Answer from the drawing. Dimensions are ordinates in mm from the lowest x, y and z of the part. A direction names the side the tool comes from. Coordinates: 2 decimals unless noted, no trailing zeros. Order: outer loops, then holes, each group sorted by start corner. A loop starts at its lowest first (then second) coordinate and runs counter-clockwise, first axis right, second up. Notation, with made-up numbers: M 84,11 L 112,11 A7 ccw 112,23 Z; hole C 32.5,-0.5 d3. An arc over 180 degrees is marked long. Write each question's results on one line, items separated by ' | '.
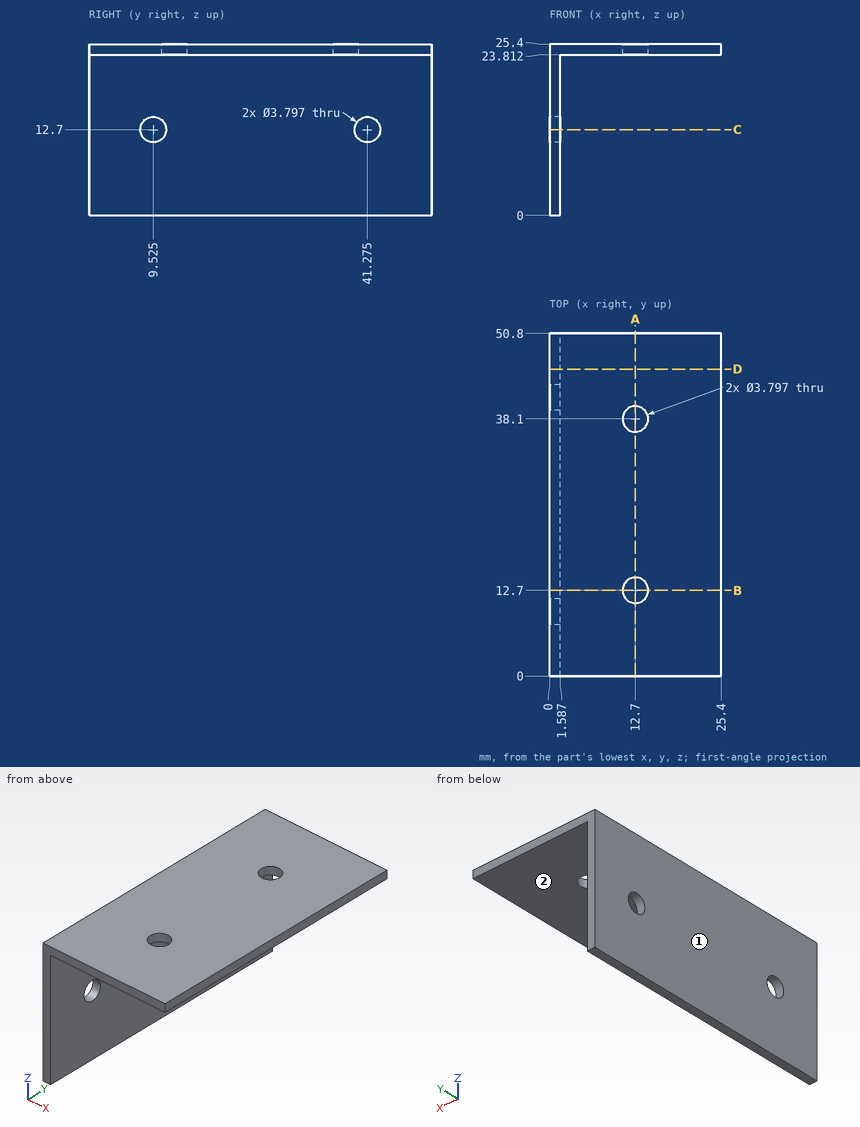
(1) The part is cut by section B-B, the plane y = 12.7. Write down the section's boundary in (x, z).
Conclusion:
outline: M 0,0 L 1.59,0 L 1.59,23.81 L 10.8,23.81 L 10.8,25.4 L 0,25.4 Z; M 14.6,23.81 L 25.4,23.81 L 25.4,25.4 L 14.6,25.4 Z
(2) The part is cut by section D-D, the plane y = 45.5. Write down the section's boundary in (x, z).
Conclusion:
outline: M 0,0 L 1.59,0 L 1.59,23.81 L 25.4,23.81 L 25.4,25.4 L 0,25.4 Z
(3) Given pin 1 (3.5 mm diameter, centred on y = 41.275, z = 12.7, fed in from -X); pin 2 (7 mm diameter, centred on y = 36.5, z = 17, fed in from +X), each flat-ended and moving along its own axis, determine where each tip first touches the part or whether it passes through.
Conclusion:
pin 1: through | pin 2: x = 1.59
(4) For the marked faces 1 and 2, determine the directions among +Z, -Z, +X, -X, +Y, -Y from which every point of the face is accessible in a straight line to the end or side of a thin tool.
Conclusion:
face 1: +Z, -Z, -X, +Y, -Y | face 2: -Z, +X, +Y, -Y
(5) Straight lines are drawn through the part: line 1 (Y direction, x = 0.95, z = 12.7); line 2 (Y direction, x = 12.7, z = 24.4); line 3 (X direction, y = 2.5, z = 17). For each, find the intervals that lie inside material, in ascending order.
Conclusion:
line 1: 0 to 7.63, 11.42 to 39.38, 43.17 to 50.8 | line 2: 0 to 10.8, 14.6 to 36.2, 40 to 50.8 | line 3: 0 to 1.59
(6) The part is cut by section A-A, the plane x = 12.7. Write down the section's boundary in (y, z).
Conclusion:
outline: M 0,23.81 L 10.8,23.81 L 10.8,25.4 L 0,25.4 Z; M 14.6,23.81 L 36.2,23.81 L 36.2,25.4 L 14.6,25.4 Z; M 40,23.81 L 50.8,23.81 L 50.8,25.4 L 40,25.4 Z
(7) The part is cut by section C-C, the plane z = 12.7. Write down the section's boundary in (x, y).
Conclusion:
outline: M 0,0 L 1.59,0 L 1.59,7.63 L 0,7.63 Z; M 0,11.42 L 1.59,11.42 L 1.59,39.38 L 0,39.38 Z; M 0,43.17 L 1.59,43.17 L 1.59,50.8 L 0,50.8 Z
